```python
from build123d import *

# Parameters (mm, degrees)
F0_R     = 14.75
F1_DEPTH = 0.25
F3_D     = 0.2
F3_DEPTH = 5
F3_TIP   = 0.0600860619


with BuildPart() as f1:
    # F0 (on Top) → F1 (new body, symmetric)
    with BuildSketch(Plane.XY):
        Circle(F0_R)
    extrude(amount=F1_DEPTH, both=True)

    # F3
    with Locations(Plane.XY.offset(0.25)):
        with Locations((12, -12), (6, -9), (6, 0), (9, 3), (0, 12), (-6, 3), (-6, -12), (-12, -6), (6, 12), (-12, -12), (12, 3), (-6, 12), (3, 6), (0, 9), (12, 9), (-12, 6), (-9, -9), (9, 0), (9, -6), (6, 3), (0, 3), (-6, 6), (6, -12), (-6, 0), (-9, 3), (-12, 9), (9, 6), (3, -3), (3, -12), (-12, 12), (6, 6), (3, -6), (12, 0), (-9, -6), (0, 6), (12, 12), (3, 9), (12, -3), (-3, -3), (-12, -3), (3, 3), (-3, -12), (-12, -9), (-3, 3), (-12, 3), (-3, 12), (12, 6), (3, 0), (3, -9), (9, -12), (-6, -9), (0, -9), (-9, 9), (9, 9), (6, -3), (-3, 0), (0, -3), (0, 0), (-9, 6), (-9, 0), (3, 12), (12, -6), (-3, -6), (-6, -3), (0, -12), (-6, 9), (9, 12), (9, -3), (12, -9), (-3, 6), (-12, 0), (0, -6), (-3, -9), (-9, -12), (-6, -6), (-9, -3), (-3, 9), (-9, 12), (6, 9), (6, -6), (9, -9)):
            Hole(F3_D / 2, depth=F3_DEPTH)
            with Locations((0, 0, -(F3_DEPTH + F3_TIP / 2))):  # 118° drill point
                Cone(0, F3_D / 2, F3_TIP, mode=Mode.SUBTRACT)


solid = f1.part
```
Here's how the part is built. I have some questions about the finished solid (model axes, mm). Round coordinates to 2 decimals unless told otherwise and drop trailing zeros. Write each loop counter-clockwise with the first axis right and the second up, starting at its lowest first coordinate (ties: lowest second). Pieces come first, ordered by that corner, then holes.
Q1. If we section it at B-B on y = 7.25: Write out the boundary of the cut face in (x, z).
Q2. Please list where these lines run through material, in increasing order: probe 1 along Y at (x, z) = (-3.5, -0.2); probe 2 along Y at (x, z) = (9.5, 0.2); probe 3 along X at (y, z) = (-4.25, -0.2).
Q3. If we section it at C-C on x = -12.5: Write out the boundary of the cut face in (y, z).
Q4. If we section it at A-A on z = 0.15: Give the number of separate pieces and of enclosed holes in the cut face, plus the area to 3 significant figures.
Answer below:
1. outline: (-12.85, -0.25) - (12.85, -0.25) - (12.85, 0.25) - (-12.85, 0.25) - close
2. probe 1: y = -14.33 to 14.33
2. probe 2: y = -11.28 to 11.28
2. probe 3: x = -14.12 to 14.12
3. outline: (-7.83, -0.25) - (7.83, -0.25) - (7.83, 0.25) - (-7.83, 0.25) - close
4. separate pieces: 1
4. enclosed holes: 69
4. area: 681 mm2
